```python
from build123d import *

# Parameters (mm, degrees)
SKETCH1_R           = 37
BOSS_EXTRUDE1_DEPTH = 10
SKETCH2_R           = 37
BOSS_EXTRUDE2_DEPTH = 10
BOSS_EXTRUDE3_REACH = 179.871
SKETCH4_W           = 10
SKETCH4_H           = 10
CUT_EXTRUDE1_DEPTH  = 188.451327016
SKETCH5_R           = 0.6
CUT_EXTRUDE2_DEPTH  = 19.75
SKETCH7_R           = 0.6
CUT_EXTRUDE4_DEPTH  = 19.75


with BuildPart() as part:
    # Sketch1 → Boss-Extrude1 (new body)
    with BuildSketch(Plane(origin=(0, 0, 0), x_dir=(1, 0, 0), z_dir=(0, 1, 0))):
        with Locations(Location((0, 0, 0), (0, 0, 270))):
            Circle(SKETCH1_R)
    extrude(amount=BOSS_EXTRUDE1_DEPTH)


with BuildPart() as body_2:
    # Sketch2 → Boss-Extrude2 (new body)
    with BuildSketch(Plane(origin=(0, 180, 0), x_dir=(1, 0, 0), z_dir=(0, 1, 0))):
        with Locations(Location((0, 0, 0), (0, 0, 270))):
            Circle(SKETCH2_R)
    extrude(amount=-BOSS_EXTRUDE2_DEPTH)

    # Sketch3 → Boss-Extrude3 (add, up to next)
    with BuildSketch(Plane(origin=(0, 10, 0), x_dir=(1, 0, 0), z_dir=(0, 1, 0)), mode=Mode.PRIVATE) as boss_extrude3_sk1:
        with BuildLine():
            Line((36.66060556, 5), (-36.66060556, 5))
            ThreePointArc((-36.66060556, 5), (-37, 0), (-36.66060556, -5))
            Line((-36.66060556, -5), (36.66060556, -5))
            ThreePointArc((36.66060556, -5), (37, 0), (36.66060556, 5))
        make_face()
    boss_extrude3_tool1 = extrude(boss_extrude3_sk1.sketch, amount=BOSS_EXTRUDE3_REACH, mode=Mode.PRIVATE) - body_2.part

    add(part.part)  # Boss-Extrude3 merges part
    add(boss_extrude3_tool1.solids().sort_by_distance((0, 10, 0))[0])

    # Sketch4 → Cut-Extrude1 (cut, through all)
    with BuildSketch(Plane(origin=(0, 180, 0), x_dir=(1, 0, 0), z_dir=(0, 1, 0))):
        with Locations((0, 37)):
            Rectangle(SKETCH4_W, SKETCH4_H)
        with Locations((0, -37)):
            Rectangle(SKETCH4_W, SKETCH4_H)
    extrude(amount=-CUT_EXTRUDE1_DEPTH, mode=Mode.SUBTRACT)

    # Sketch5 → Cut-Extrude2 (cut)
    with BuildSketch(Plane(origin=(0, 180, 0), x_dir=(1, 0, 0), z_dir=(0, 1, 0))):
        with Locations(Location((-18.5, 0, 0), (0, 0, 270))):
            Circle(SKETCH5_R)
        with Locations(Location((0, 0, 0), (0, 0, 270))):
            Circle(SKETCH5_R)
        with Locations(Location((18.5, 0, 0), (0, 0, 270))):
            Circle(SKETCH5_R)
    extrude(amount=-CUT_EXTRUDE2_DEPTH, mode=Mode.SUBTRACT)

    # Sketch7 → Cut-Extrude4 (cut)
    with BuildSketch(Plane.XZ):
        with Locations(Location((-19.25, 0, 0), (0, 0, 270))):
            Circle(SKETCH7_R)
        with Locations(Location((0, 0, 0), (0, 0, 90))):
            Circle(SKETCH7_R)
        with Locations(Location((19.25, 0, 0), (0, 0, 270))):
            Circle(SKETCH7_R)
    extrude(amount=-CUT_EXTRUDE4_DEPTH, mode=Mode.SUBTRACT)


solid = body_2.part
```
Geometry check sheet. Reference: the model listing, model coordinates, mm. A direction names the side the tool comes from. Give positions to 0.01 mm unless a question says otherwise; leave off trailing zeros. Write each loop counter-clockwise with the first axis right and the second up, starting at its lowest first coordinate (ties: lowest second). Pieces come first, ordered by that corner, then holes.
1) Section check D-D, the plane z = -18.5. Record the boundary of the cut face in (x, y).
2) Section check B-B, the plane x = 26.5. Record the boundary of the cut face in (y, z).
3) Gauge pin test, flat ends, axial feed: pin 1 (3.5 mm diameter, centred on y = 176, z = -35, fed in from +X); pin 2 (1.4 mm diameter, centred on y = 173.5, z = 34.5, fed in from -X); pin 3 (5 mm diameter, centred on y = 175, z = -34.5, fed in from -X). Record the tip position at first contact, or that the pin passes through.
4) Release check for a two-part mould opening along Y. For faces 1 (the flat face through (5, 175, -34)), 2 (the flat face through (1, 0, -1)), 3 (the flat face through (-1, 89, 5)) record: pulls with the +Y half, pulls with the -Y half, needs draft (parallel to the pull), parting line crosses it, or undercut.
5) Material ranges on L1, parallel to Y at x = 31, z = 11; L2, parallel to Z at x = 16, y = 15; L3, parallel to Z at x = 19, y = 12, recorded low to high.
6) Section check A-A, the plane z = -27. Record the boundary of the cut face in (x, y), and give its area (3 significant figures).
7) Access from +Z, -Z, +X, -X, +Y, -Y to the whole of each face (thin tool, end or side, straight path). Record for faces 4 (the flat face through (5, 5, 34)), 5 (the flat face through (0, 5, -32)), 6 (the flat face through (1, 170, 17)).
8) Section check C-C, the plane y = 51. Record the boundary of the cut face in (x, z), and give its area (3 significant figures).
Computed:
1. outline: (-32.04, 0) - (32.04, 0) - (32.04, 10) - (-32.04, 10) - close; (-32.04, 170) - (32.04, 170) - (32.04, 180) - (-32.04, 180) - close
2. outline: (0, -25.82) - (10, -25.82) - (10, -5) - (170, -5) - (170, -25.82) - (180, -25.82) - (180, 25.82) - (170, 25.82) - (170, 5) - (10, 5) - (10, 25.82) - (0, 25.82) - close
3. pin 1: stops at x = 16.23
3. pin 2: stops at x = -15.05
3. pin 3: stops at x = -18.57
4. face 1: needs draft
4. face 2: pulls with the -Y half
4. face 3: undercut
5. L1: y = 0 to 10, 170 to 180
5. L2: z = -5 to 5
5. L3: z = -5 to -0.55, 0.55 to 5
6. outline: (-25.3, 0) - (25.3, 0) - (25.3, 10) - (-25.3, 10) - close; (-25.3, 170) - (25.3, 170) - (25.3, 180) - (-25.3, 180) - close
6. area: 1,010 mm2
7. face 4: +Z, +Y, -Y
7. face 5: -Z, +Y, -Y
7. face 6: +Z, +X, -X
8. outline: (-36.66, -5) - (36.66, -5) arc R37 ccw to (36.66, 5) - (-36.66, 5) arc R37 ccw to start
8. area: 738 mm2
